Job drawing, mm, ordinate dimensions from the low corner. One solid piece. A direction names the side the tool comes from. Round coordinates to 2 decimals unless told otherwise and drop trailing zeros.
1) Mould opens along X. For the marked faces 3, 4 and 5 say: +X half, -X half, draft (parallel to the pull), parting line (faces both ways), or undercut.
2) Probe line 1 (X direction, y = 6, z = 12) (1 decimal); line 2 (Y direction, x = 29.5, z = 5.5) (1 decimal); line 3 (X direction, y = 20, z = 13.75) (1 decimal). List the from-to ranges inside material, lowest first.
3) Drop flat-ended pins along their axis: P1, Ø2, axis at x = 22, z = 4, coming from the +Y side; P2, Ø1.5, axis at y = 26, z = 3.5, coming from the -X side (1 decimal); P3, Ø3, axis at y = 15, z = 7, coming from the -X side. Give the stop position or say it passes through.
4) 3-axis set-ups, long thin cutter, end or side, ignore diameter. For the marked faces 1 and 2: which of +Z, -Z, +X, -X, +Y, -Y reach the whole face in a straight line?
5) Band-saw the part on A-A, the plane z = 10.25. State how many separate pieces and enclosed holes the cut face has, then the cut area to 3 significant figures.
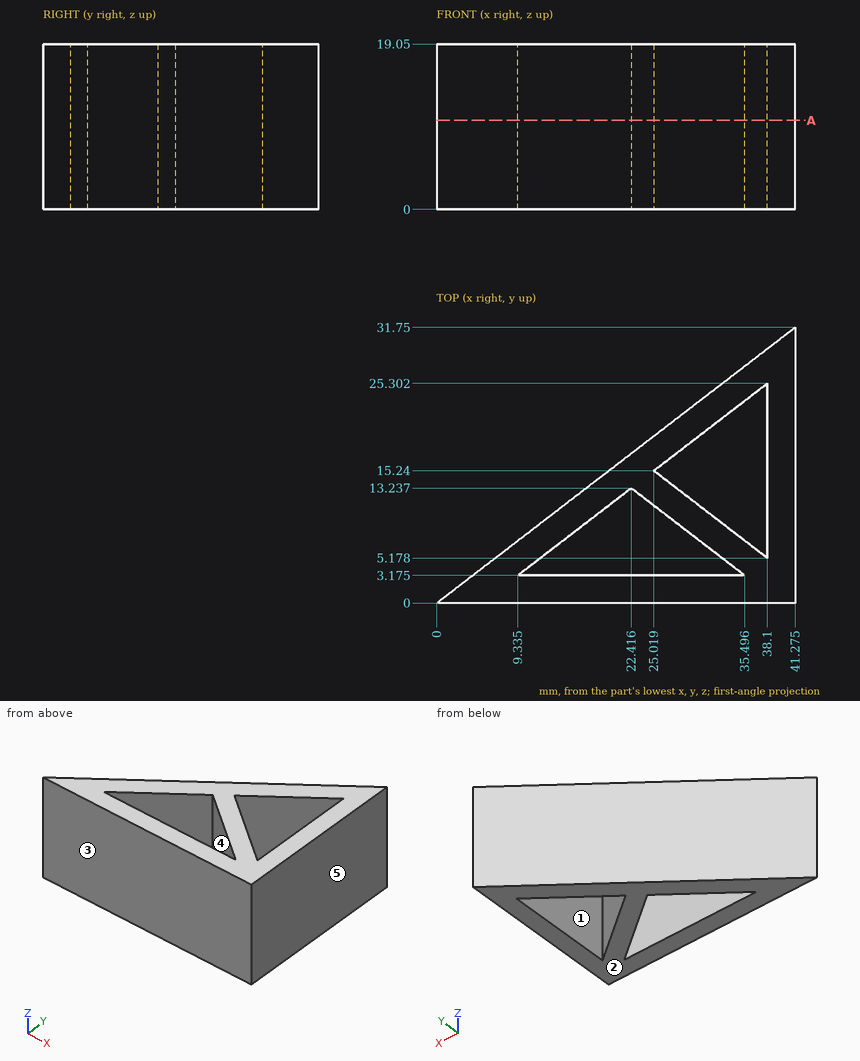
Reported:
1. face 3: draft
1. face 4: undercut
1. face 5: +X half
2. line 1: x = 7.8 to 13, 31.8 to 37, 38.1 to 41.3
2. line 2: y = 0 to 3.2, 7.8 to 11.8, 18.7 to 22.7
2. line 3: x = 26 to 31.2, 38.1 to 41.3
3. P1: stops at y = 17.69
3. P2: stops at x = 32.8
3. P3: stops at x = 17.55
4. face 1: +Z, -Z
4. face 2: -Z, +X, -X, +Y, -Y
5. separate pieces: 1
5. enclosed holes: 2
5. area: 392 mm2
